The listing builds one solid part. Answer for the finished solid, in the listing's coordinates (mm). Face numbers are marked on the shaded views. A direction names the side the tool comes from. Give positions to 0.01 mm unless a question says otherwise; leave off trailing zeros. Write each loop counter-clockwise with the first axis right and the second up, starting at its lowest first coordinate (ties: lowest second). Pieces come first, ordered by that corner, then holes. Notation, with made-up numbers: (35, -4) -> (47, -4) arc R27 ccw to (47, 21) -> close; hole circle Ø6 at (43.25, 28). An arc over 180 degrees is marked (long way). Put each result on its own line as item: value. Start each with the question number.
1) For a pull along Z with two mould halves and no side action, classify the marked faces 1, 2, 3 and 4 as released by +Z, released by -Z, zero draft, split by the parting line, or undercut.
2) A cutting plane is placed at B-B (x = -23.5). Write down the section's boundary in (y, z).
3) Flat-ended cylindrical pins translate along their axes: pin 1 Ø2 at (x, y) = (-16, 46.5) entering from +Z; pin 2 Ø1 at (y, z) = (35.5, 28) entering from -X. Find the tip coordinate at first contact, or state that the pin passes through.
4) Find the intervals of material crossed by line 1 along Y through (x, z) = (-31.25, 29.25); line 2 along Y through (x, z) = (-16.75, 23.75); line 3 along Y through (x, z) = (-33.25, 19), in increasing order. Write a range as from..to.
5) A cutting plane is placed at A-A (y = 45). Write down the section's boundary in (x, z).
6) For the marked faces 5, 6, 7, 8 and 9, determine the directions among +Z, -Z, +X, -X, +Y, -Y from which every point of the face is accessible in a straight line to the end or side of a thin tool.
7) A cutting plane is placed at D-D (y = 37). Write down the section's boundary in (x, z).
8) A cutting plane is placed at C-C (z = 18). Write down the section's boundary in (x, y), then the cut area to 3 significant figures.
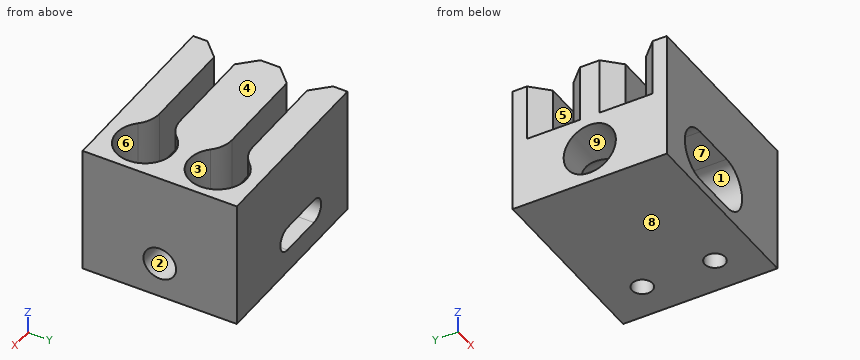
Autodesk Inventor part; units mm, degrees
ref_plane "Work Plane1" through (0, 33.012, 0) normal (0, 1, 0) x (-1, 0, 0)
ref_plane "Work Plane2" through (0, 0, 19.2509) normal (0, 0, 1) x (1, 0, 0)
ref_plane "Work Plane3" through (-21.9672, 40.562, 30.2509) normal (0, 1, 0) x (1, 0, 0)
ref_plane "Work Plane1" through (0, 33.012, 0) normal (0, 1, 0) x (-1, 0, 0)
sketch "Sketch1" plane through (0, 33.012, 0) normal (0, 1, 0) x (-1, 0, 0)
  line L0 (12.3254, 14.5509) -> (12.3254, 30.2509)
  line L1 (20.3254, 14.5509) -> (12.3254, 14.5509)
  line L2 (12.3254, 30.2509) -> (20.3254, 30.2509)
  line L3 (20.3254, 30.2509) -> (20.3254, 14.5509)
extrude "Extrusion12" add sketch "Sketch1" along normal blind 17
sketch "Sketch2" plane through (-20.3254, 33.012, 30.2509) normal (0, 0, 1) x (1, 0, 0)
  arc A0 (0.2308, 10.75) -> (0.2308, 13.25) centre (3.5, 12) ccw
  line L0 (-0.0992, 10.75) -> (-0.0992, 13.25)
  line L1 (0.2308, 10.75) -> (-0.0992, 10.75)
  line L2 (0.2308, 13.25) -> (-0.0992, 13.25)
  circle A1 centre (3.5, 12) radius 1.5
  dimension "d52" = 2.5
  dimension "d66" = 3
  dimension "d67" = 2
extrude "Extrusion11" cut sketch "Sketch2" against normal blind 7 draft 0 contours L1 L0 L2 A0 | A1
sketch "Sketch3" plane through (-20.3254, 33.012, 14.5509) normal (-1, 0, 0) x (0, 0, 1)
  line L0 (6.75, 5.0877) -> (6.75, 0)
  line L1 (1.25, 0) -> (1.25, 5.0877)
  line L2 (4, 6.6754) -> (6.75, 5.0877)
  line L3 (1.25, 5.0877) -> (4, 6.6754)
  line L4 (6.75, 0) -> (1.25, 0)
extrude "Extrusion10" cut sketch "Sketch3" against normal blind 2.5
sketch "Sketch4" plane through (0, 33.012, 0) normal (0, 1, 0) x (-1, 0, 0)
  line L0 (12.3254, 30.2509) -> (31.3754, 30.2509)
  line L1 (20.3254, 14.5509) -> (20.3254, 22.5509)
  line L2 (12.3254, 22.5509) -> (12.3254, 30.2509)
  line L3 (20.3254, 14.5509) -> (31.3754, 14.5509)
  line L4 (20.3254, 22.5509) -> (12.3254, 22.5509)
  line L5 (31.3754, 30.2509) -> (31.3754, 14.5509)
extrude "Extrusion9" cut sketch "Sketch4" along normal blind 7 draft 0
ref_plane "Work Plane2" through (0, 0, 19.2509) normal (0, 0, 1) x (1, 0, 0)
sketch "Sketch12" plane through (-20.3254, 50.012, 30.2509) normal (0, 0, 1) x (1, 0, 0)
  line L0 (0, -17) -> (0, 0)
  line L1 (0, 0) -> (-15, 0)
  line L2 (-15, 0) -> (-15, -10)
  line L3 (-15, -10) -> (0, -10)
  line L4 (0, -10) -> (0, 0)
  line L5 (0, -6.25) -> (0, -3.75)
  line L6 (0, -3.75) -> (-15, -3.75)
  line L7 (-15, -3.75) -> (-15, -6.25)
  line L8 (-15, -6.25) -> (0, -6.25)
  line L9 (0, -6.25) -> (0, -3.75)
  line L10 (0, -10) -> (8, -10)
  line L11 (8, -10) -> (8, 0)
  point P0 (20.3254, -50.012)
  point P1 (-15, -6.25)
  dimension "d44" = 23
extrude "Extrusion15" add sketch "Sketch12" against normal up to surface (15.7 mm away)
extrude "Extrusion16" cut sketch "Sketch12" against normal up to surface (7 mm away) contours L8 L2 L6 L0
sketch "Sketch6" plane through (0, 40.012, 0) normal (0, -1, 0) x (1, 0, 0)
  line L0 (-22.8754, 17.4009) -> (-28.3754, 17.4009)
  arc A0 (-28.3754, 20.4009) -> (-28.3754, 17.4009) centre (-28.3754, 18.9009) ccw
  line L1 (-28.3754, 20.4009) -> (-22.8754, 20.4009)
  arc A1 (-22.8754, 17.4009) -> (-22.8754, 20.4009) centre (-22.8754, 18.9009) ccw
extrude "Extrusion7" cut sketch "Sketch6" against normal blind 10 draft 0
sketch "Sketch7" plane through (-12.3254, 33.012, 14.5509) normal (0, 0, -1) x (-1, 0, 0)
  point P0 (4.5, 12)
hole "Hole6" at (-16.8254, 45.012, 14.5509) direction (0, 0, 1) diameter 2.5 end through all
sketch "Sketch9" plane through (-17.8254, 33.012, 14.5509) normal (-1, 0, 0) x (0, 0, 1)
  point P0 (4, 3.5)
hole "Hole4" at (-17.8254, 36.512, 18.5509) direction (1, 0, 0) diameter 3 depth 5.5
fillet "Fillet8" radius 2.5 1 edges at (-20.3254, 33.012, 21.9259)
fillet "Fillet7" radius 2.5 1 edges at (-20.3254, 33.012, 15.1759)
fillet "Fillet6" radius 3.5 1 edges at (-20.0946, 43.762, 26.7509)
fillet "Fillet5" radius 3.5 1 edges at (-20.0946, 46.262, 26.7509)
chamfer "Chamfer1" [suppressed]
chamfer "Chamfer2" distance 2 angle 45 2 edges at (-35.3254, 46.262, 26.7509) (-35.3254, 43.762, 26.7509)
sketch "Sketch14" plane through (-20.3254, 40.012, 22.5509) normal (0, 0, 1) x (1, 0, 0)
  arc A0 (0, -4.5) -> (2.5, -7) centre (2.5, -4.5) ccw
  line L0 (0, -1.9123) -> (0, -4.5)
  line L1 (0, -1.9123) -> (2.5, -1.9123)
  line L2 (2.5, -1.9123) -> (2.5, -7)
  line L3 (0, -1.9123) -> (2.5, -7)
  arc A1 (0, -4.5) -> (2.5, -7) centre (2.5, -4.5) ccw
  point P0 (20.3254, -40.012)
  point P1 (2.5, -7)
extrude "Extrusion18" cut sketch "Sketch14" against normal blind 1.3875 contours L0 L3 A0
ref_plane "Work Plane3" through (-21.9672, 40.562, 30.2509) normal (0, 1, 0) x (1, 0, 0)
sketch "Sketch15" plane through (0, 33.012, 0) normal (0, -1, 0) x (1, 0, 0)
  line L0 (-25.3064, 10.3119) -> (-9.5646, 10.3119)
  line L1 (-9.5646, 10.3119) -> (-9.5646, 26.9005)
  line L2 (-9.5646, 26.9005) -> (-25.3064, 26.9005)
  line L3 (-25.3064, 26.9005) -> (-25.3064, 10.3119)
  point P0 (0, 0)
extrude "Extrusion19" cut sketch "Sketch15" against normal up to surface (7 mm away)
mirror "Mirror1" about plane through (-21.9672, 40.562, 30.2509) normal (0, 1, 0)
sketch "Sketch16" plane through (-35.3254, 31.112, 30.2509) normal (0, -1, 0) x (1, 0, 0)
  line L0 (0, 0) -> (0, -15.7)
  line L1 (23, -15.7) -> (0, -15.7)
  line L2 (23, 0) -> (23, -15.7)
  line L3 (23, 0) -> (0, 0)
  arc A0 (12.45, -12.85) -> (12.45, -9.85) centre (12.45, -11.35) ccw
  line L4 (6.95, -12.85) -> (12.45, -12.85)
  arc A1 (6.95, -9.85) -> (6.95, -12.85) centre (6.95, -11.35) ccw
  line L5 (12.45, -9.85) -> (6.95, -9.85)
  arc A2 (12.45, -14.55) -> (12.45, -8.15) centre (12.45, -11.35) ccw
  line L6 (12.45, -14.55) -> (6.95, -14.55)
  arc A3 (6.95, -8.15) -> (6.95, -14.55) centre (6.95, -11.35) ccw
  line L7 (6.95, -8.15) -> (12.45, -8.15)
  point P0 (35.3254, -30.2509)
  dimension "d71" = 3.2
extrude "Extrusion20" cut sketch "Sketch16" against normal blind 15 contours L6 A3 L7 A2
sketch "Sketch18" plane through (-12.3254, 50.012, 30.2509) normal (1, 0, 0) x (0, 0, -1)
  circle A0 centre (11.35, -9.45) radius 2
  line L0 (15.7, -18.9) -> (15.7, 0)
  line L1 (15.7, -9.45) -> (7, -9.45) construction
  line L2 (7, -8.5) -> (7, -1.5)
  line L3 (7, -10.4) -> (7, -17.4)
  point P0 (30.2509, -50.012)
  point P1 (7, -2.625)
  point P2 (7, -7.375)
  point P3 (7, -16.275)
  point P4 (7, -11.525)
  dimension "d78" = 4
extrude "Extrusion22" cut sketch "Sketch18" against normal blind 5.7
sketch "Sketch19" plane through (-18.0254, 40.562, 18.9009) normal (1, 0, 0) x (0, 0, -1)
  circle A0 centre (0, 0) radius 2
  circle A1 centre (0, 0) radius 1.5
  point P0 (18.9009, -40.562)
  dimension "d81" = 3
extrude "Extrusion23" cut sketch "Sketch19" against normal blind 6.3625 contours A1
sketch "Sketch20" plane through (-35.3254, 41.762, 23.2509) normal (-1, 0, 0) x (0, 0, 1)
  circle A0 centre (-4.35, -1.2) radius 3.2
  circle A1 centre (-4.35, -1.2) radius 1.5
  line L0 (-7.55, -10.65) -> (-7.55, 4.35)
  line L1 (-1.15, -10.65) -> (-1.15, 4.35)
  point P0 (-23.2509, -41.762)
extrude "Extrusion24" cut sketch "Sketch20" against normal blind 6.3625 contours A0 | A1
Reply:
1. face 1: undercut
1. face 2: undercut
1. face 3: zero draft
1. face 4: released by +Z
2. outline: (31.11, 14.55) -> (50.01, 14.55) -> (50.01, 17.4) -> (46.11, 17.4) -> (46.11, 15.7) -> (31.11, 15.7) -> close; (31.11, 22.1) -> (46.11, 22.1) -> (46.11, 20.4) -> (50.01, 20.4) -> (50.01, 30.25) -> (46.26, 30.25) -> (46.26, 23.25) -> (43.76, 23.25) -> (43.76, 30.25) -> (37.36, 30.25) -> (37.36, 23.25) -> (34.86, 23.25) -> (34.86, 30.25) -> (31.11, 30.25) -> close
3. pin 1: stops at z = 23.25
3. pin 2: stops at x = -13.51
4. line 1: y = 31.11..34.86, 37.36..43.76, 46.26..50.01
4. line 2: y = 31.11..32.61, 39.61..41.51, 48.51..50.01
4. line 3: y = 31.11..37.36, 43.76..50.01
5. outline: (-35.33, 14.55) -> (-18.08, 14.55) -> (-18.08, 23.25) -> (-35.33, 23.25) -> close; (-15.58, 14.55) -> (-12.33, 14.55) -> (-12.33, 30.25) -> (-13.33, 30.25) -> (-13.33, 23.25) -> (-15.58, 23.25) -> close; hole (-28.38, 15.7) -> (-22.88, 15.7) arc R3.2 ccw to (-22.88, 22.1) -> (-28.38, 22.1) arc R3.2 ccw to start
6. face 5: +Z, -X
6. face 6: +Z
6. face 7: -Y
6. face 8: -Z, +X, -X, +Y, -Y
6. face 9: -X
7. outline: (-35.33, 14.55) -> (-17.71, 14.55) -> (-17.71, 23.25) -> (-35.33, 23.25) -> close; (-15.95, 14.55) -> (-12.33, 14.55) -> (-12.33, 30.25) -> (-13.44, 30.25) -> (-13.44, 23.25) -> (-15.95, 23.25) -> close; hole (-28.38, 15.7) -> (-22.88, 15.7) arc R3.2 ccw to (-22.88, 22.1) -> (-28.38, 22.1) arc R3.2 ccw to start
8. outline: (-35.33, 31.11) -> (-31.45, 31.11) -> (-31.45, 37.49) -> (-35.33, 37.49) -> close; (-35.33, 43.63) -> (-31.45, 43.63) -> (-31.45, 46.11) -> (-29.57, 46.11) -> (-29.57, 50.01) -> (-35.33, 50.01) -> close; (-21.68, 46.11) -> (-19.8, 46.11) -> (-19.8, 41.76) -> (-18.03, 41.76) -> (-18.03, 42.35) -> (-12.33, 42.35) -> (-12.33, 50.01) -> (-21.68, 50.01) -> close; (-19.8, 31.11) -> (-12.33, 31.11) -> (-12.33, 38.78) -> (-18.03, 38.78) -> (-18.03, 39.36) -> (-19.8, 39.36) -> close; hole circle Ø2.5 at (-16.83, 36.11); hole circle Ø2.5 at (-16.83, 45.01)
8. area: 171 mm2
